from build123d import *

# Parameters (mm, degrees)
BOX_W                  = 10
BOX_H                  = 20
BOX_DEPTH              = 10
BOX001_W               = 7.07
BOX001_H               = 20
BOX001_DEPTH           = 7.07
BOX001_PLACEMENT_ANGLE = 45


with BuildPart() as cubo:
    # Box → Box (new body)
    with BuildSketch(Plane.XY):
        with Locations((5, 10)):
            Rectangle(BOX_W, BOX_H)
    extrude(amount=BOX_DEPTH)


with BuildPart() as fusion:
    # Box001 → Box001 (new body)
    with BuildSketch(Plane.XY):
        with Locations((3.535, 10)):
            Rectangle(BOX001_W, BOX001_H)
    extrude(amount=BOX001_DEPTH)


with BuildPart() as fusion_1:
    # Box001 placement: moved
    add(fusion.part.moved(Location((-0.004245, 0, 9.965))).rotate(Axis((-0.004245, 0, 9.965), (0, 1, 0)), BOX001_PLACEMENT_ANGLE))

    # Fusion: union Cubo
    add(cubo.part)


solid = fusion_1.part
Part model, mm, in its own coordinate system. Coordinates: 2 decimals unless noted, no trailing zeros. Order: outer loops, then holes, each group sorted by start corner. A loop starts at its lowest first (then second) coordinate and runs counter-clockwise, first axis right, second up. Notation, with made-up numbers: M 46.5,-25.5 L 59.5,-25.5 A11 cw 59.5,-11.5 Z; hole C 65.5,24 d8. An arc over 180 degrees is marked long. Use a Markdown table: item, result.
(1) Cut at B-B on x = 4.25. Write the cut outline in (y, z).
A:
| item | result |
|---|---|
| outline | M 0,0 L 20,0 L 20,14.22 L 0,14.22 Z |
(2) Cut at C-C on z = 12.75. Write the cut outline in (x, y).
A:
| item | result |
|---|---|
| outline | M 2.78,0 L 7.21,0 L 7.21,20 L 2.78,20 Z |
(3) Flat gauge pins, fed straight in: pin 1 (5 mm diameter, centred on y = 10, z = 5.5, fed in from -X); pin 2 (3 mm diameter, centred on x = 6, y = 4, fed in from +Z). Where does each tip first touch, or does it go through?
A:
| item | result |
|---|---|
| pin 1 | stops at x = 0 |
| pin 2 | stops at z = 14.96 |
(4) Cut at A-A on y = 3.25. Write the cut outline in (x, z) (3 decimals).
A:
| item | result |
|---|---|
| outline | M -0.004,9.965 L 0,9.961 L 0,0 L 10,0 L 10,10 L 9.959,10 L 4.995,14.964 L 0.031,10 L 0,10 L 0,9.969 Z |
(5) Probe L1, parallel to X at y = 6.5, z = 6; L2, parallel to Z at x = 2, y = 14.75; L3, parallel to Z at x = 1.25, y = 17. List the from-to ranges inside material, lowest first.
A:
| item | result |
|---|---|
| L1 | x = 0 to 10 |
| L2 | z = 0 to 11.97 |
| L3 | z = 0 to 11.22 |
